Source: CAD feature listing. Evaluate the final solid. Frame: model axes, mm. A direction names the side the tool comes from. Round coordinates to 2 decimals unless told otherwise and drop trailing zeros. Write each loop counter-clockwise with the first axis right and the second up, starting at its lowest first coordinate (ties: lowest second). Pieces come first, ordered by that corner, then holes. Notation, with made-up numbers: M -31,16 L -22,16 A22 cw -22,55 Z; hole C -10,-29 d9. An arc over 180 degrees is marked long. Use a Markdown table: item, result.
```python
from build123d import *

# Parameters (mm, degrees)
F0_R     = 14.5
F0_R_2   = 9.5
F1_DEPTH = 20
F2_W     = 17
F2_H     = 20.348274
F3_DEPTH = 20
F5_DEPTH = 15
F6_W     = 7.194839
F6_H     = 10
F7_DEPTH = 5


with BuildPart() as f1:
    # F0 (on Top) → F1 (new body)
    with BuildSketch(Plane.XY):
        Circle(F0_R)
        Circle(F0_R_2, mode=Mode.SUBTRACT)
    extrude(amount=F1_DEPTH)

    # F2 (on Top) → F3 (cut)
    with BuildSketch(Plane.XY):
        with Locations((0, -10.174137)):
            Rectangle(F2_W, F2_H)
    extrude(amount=F3_DEPTH, mode=Mode.SUBTRACT)

    # F4 (on face) → F5 (join)
    with BuildSketch(Plane(origin=(0, 0, 0), x_dir=(1, 0, 0), z_dir=(0, 0, -1))):
        with BuildLine():
            ThreePointArc((-14.282857, -2.5), (-14.5, 0), (-14.282857, 2.5))
            Line((-14.282857, 2.5), (-26.692857, 2.5))
            Line((-26.692857, 2.5), (-26.692857, -2.5))
            Line((-26.692857, -2.5), (-14.282857, -2.5))
        make_face()
    extrude(amount=-F5_DEPTH)

    # F6 (on face) → F7 (cut)
    with BuildSketch(Plane.XZ.offset(2.5)):
        with Locations((-18.09742, 10)):
            Rectangle(F6_W, F6_H)
    extrude(amount=-F7_DEPTH, mode=Mode.SUBTRACT)


solid = f1.part
```
Q1. Section C-C on z = 4.5. Return loops of the section in (x, y), plus the area to 3 significant figures.
Results are:
| item | result |
|---|---|
| outline | M -26.69,-2.5 L -14.28,-2.5 A14.5 ccw -8.5,-11.75 L -8.5,-4.24 A9.5 cw long 8.5,-4.24 L 8.5,-11.75 A14.5 ccw long -14.28,2.5 L -26.69,2.5 Z |
| area | 343 mm^2 |
Q2. Section A-A on z = 7.75. Return loops of the section in (x, y), plus the area to 3 significant figures.
Results are:
| item | result |
|---|---|
| outline | M -26.69,-2.5 L -21.69,-2.5 L -21.69,2.5 L -26.69,2.5 Z; M -14.5,-2.5 L -14.28,-2.5 A14.5 ccw -8.5,-11.75 L -8.5,-4.24 A9.5 cw long 8.5,-4.24 L 8.5,-11.75 A14.5 ccw long -14.28,2.5 L -14.5,2.5 Z |
| area | 307 mm^2 |
Q3. Section B-B on y = -3.5. Return loops of the section in (x, z).
Results are:
| item | result |
|---|---|
| outline | M -14.07,0 L -8.83,0 L -8.83,20 L -14.07,20 Z; M 8.83,0 L 14.07,0 L 14.07,20 L 8.83,20 Z |
Q4. Reachability of faces 1 (the flat face through (-24, 0, 15)), 2 (the flat face through (-22, -2.5, 6)), 3 (the flat face through (-14.5, 0, 10)) from +Z, -Z, +X, -X, +Y, -Y: full face, straight path, thin tool, end or side. Return the list, or none.
Results are:
| item | result |
|---|---|
| face 1 | +Z, -X, +Y, -Y |
| face 2 | +Z, -Z, -X, -Y |
| face 3 | +Z, +Y, -Y |
Q5. Line query: L1, parallel to X at y = 0, z = 6.75; L2, parallel to X at y = 8.5, z = 14.5; L3, parallel to X at y = 8.75, z = 9. Output: solid intervals per line, ascending.
Results are:
| item | result |
|---|---|
| L1 | -26.69 to -21.69, -14.5 to -9.5, 9.5 to 14.5 |
| L2 | -11.75 to -4.24, 4.24 to 11.75 |
| L3 | -11.56 to -3.7, 3.7 to 11.56 |
Q6. Section D-D on x = -19.5. Return loops of the section in (y, z).
Results are:
| item | result |
|---|---|
| outline | M -2.5,0 L 2.5,0 L 2.5,5 L -2.5,5 Z |
Q7. First-contact query: pin 1 Ø6 at (x, z) = (-18.5, 6) entering from -Y; pin 2 Ø2 at (y, z) = (-6.5, 18) entering from -X; pin 3 Ø12 at (y, z) = (7.5, 16.5) entering from +X; pin 4 Ø2 at (x, z) = (-18.5, 7.5) entering from +Y. Flat tips, straight axial feed; report the tip coordinate or a pass-through.
Results are:
| item | result |
|---|---|
| pin 1 | y = -2.5 |
| pin 2 | x = -13.42 |
| pin 3 | x = 14.42 |
| pin 4 | through |
Q8. Mould query, pull axis Y, two halves, no side actions, for faces 4 (the flat face through (-26.693, 0, 7)), 5 (the cylindrical face through (0.27, 9.496, 9.86)), 6 (the flat face through (-22, 2.5, 6)). Classes: +Y half, -Y half, draft (parallel to the pull), parting line (faces both ways), or undercut.
Results are:
| item | result |
|---|---|
| face 4 | draft |
| face 5 | undercut |
| face 6 | +Y half |
